from build123d import *

# Parameters (mm, degrees)
F1_W          = 62.5
F1_H          = 102.5
F1_W_2        = 57.5
F1_H_2        = 97.5
F2_DEPTH      = 37
F3_W          = 62.5
F3_H          = 102.5
F4_DEPTH      = 2.5
F6_DEPTH      = 2.501
F7_W          = 51
F7_H          = 72
F8_DEPTH      = 1.2
F10_DEPTH     = 2.5
F11_R         = 1.75
F12_DEPTH     = 102.501
F13_T1_DEPTH  = 42.5
F13_T3_DEPTH  = 57.5
F13_T5_DEPTH  = 42.5
F13_T7_DEPTH  = 57.5
F13_T9_DEPTH  = 44.4614347816
F13_T11_DEPTH = 57.9568101466
F13_T13_DEPTH = 40.0817550719
F13_T15_DEPTH = 127.5
F13_T17_DEPTH = 87.5
F14_R         = 1


# Not quite as in the source:
# - a fillet or chamfer that OpenCascade refuses, or shapes differently, is made with other operations: its cross-section is extruded or revolved along the edge and cut away or added


with BuildPart() as f2:
    # F1 (on Top) → F2 (new body)
    with BuildSketch(Plane.XY):
        with Locations((28.75, 48.75)):
            Rectangle(F1_W, F1_H)
        with Locations((28.75, 48.75)):
            Rectangle(F1_W_2, F1_H_2, mode=Mode.SUBTRACT)
    extrude(amount=F2_DEPTH)

    # F3 (on Top) → F4 (join)
    with BuildSketch(Plane.XY):
        with Locations((28.75, 48.75)):
            Rectangle(F3_W, F3_H)
    extrude(amount=F4_DEPTH)

    # F5 (on face) → F6 (cut, through all)
    with BuildSketch(Plane.XY.offset(2.5)):
        with BuildLine():
            ThreePointArc((17.25, 90.5), (16.25, 89.5), (17.25, 88.5))
            Line((17.25, 88.5), (40.25, 88.5))
            ThreePointArc((40.25, 88.5), (41.25, 89.5), (40.25, 90.5))
            Line((40.25, 90.5), (17.25, 90.5))
        make_face()
        with BuildLine():
            ThreePointArc((17.25, 13), (16.25, 12), (17.25, 11))
            Line((17.25, 11), (40.25, 11))
            ThreePointArc((40.25, 11), (41.25, 12), (40.25, 13))
            Line((40.25, 13), (17.25, 13))
        make_face()
    extrude(amount=-F6_DEPTH, mode=Mode.SUBTRACT)

    # F7 (on face) → F8 (cut)
    with BuildSketch(Plane(origin=(0, 0, 0), x_dir=(1, 0, 0), z_dir=(0, 0, -1))):
        with Locations((28.75, -53.5)):
            Rectangle(F7_W, F7_H)
    extrude(amount=-F8_DEPTH, mode=Mode.SUBTRACT)

    # F9 (on face) → F10 (join)
    with BuildSketch(Plane.XY.offset(2.5)):
        Polygon((0, 32.5), (0, 30), (28.5635979803, 46.412179039), (26.5233409817, 47.7398805363), align=None)
        Polygon((26.5233409817, 47.7398805363), (28.5635979803, 46.412179039), (30.6038549789, 47.5844775418), (28.5635979803, 48.912179039), align=None)
        Polygon((30.6038549789, 47.5844775418), (28.5635979803, 46.412179039), (57.5, 27.5817550719), (57.5, 30.0817550719), align=None)
        Polygon((28.5635979803, 48.912179039), (30.6038549789, 47.5844775418), (57.5, 63.0385652184), (57.5, 65.5385652184), align=None)
        Polygon((0, 65), (26.5233409817, 47.7398805363), (28.5635979803, 48.912179039), (0, 67.5), align=None)
    extrude(amount=F10_DEPTH)

    # F11 (on face) → F12 (cut, through all)
    with BuildSketch(Plane(origin=(0, 100, 0), x_dir=(-1, 0, 0), z_dir=(0, 1, 0))):
        with Locations((-14.5, 29.5)):
            Circle(F11_R)
        with Locations((-43, 29.5)):
            Circle(F11_R)
    extrude(amount=-F12_DEPTH, mode=Mode.SUBTRACT)

    # F13: fillet of radius 5 on 12 edges, made by hand

    # F13_s2 → F13_t1 (join)
    with BuildSketch(Plane.XZ.offset(-42.5)):
        with BuildLine():
            ThreePointArc((0, 7.5), (1.4644660941, 3.9644660941), (5, 2.5))
            Line((5, 2.5), (0, 2.5))
            Line((0, 2.5), (0, 7.5))
        make_face()
    extrude(amount=F13_T1_DEPTH)

    # F13_s4 → F13_t3 (join)
    with BuildSketch(Plane.XZ.offset(-77.5)):
        with BuildLine():
            ThreePointArc((0, 7.5), (1.4644660941, 3.9644660941), (5, 2.5))
            Line((5, 2.5), (0, 2.5))
            Line((0, 2.5), (0, 7.5))
        make_face()
    extrude(amount=F13_T3_DEPTH)

    # F13_s6 → F13_t5 (join)
    with BuildSketch(Plane.XZ.offset(-97.5)):
        with BuildLine():
            ThreePointArc((0, 7.5), (1.4644660941, 3.9644660941), (5, 2.5))
            Line((5, 2.5), (0, 2.5))
            Line((0, 2.5), (0, 7.5))
        make_face()
    extrude(amount=F13_T5_DEPTH)

    # F13_s8 → F13_t7 (join)
    with BuildSketch(Plane.YZ):
        with BuildLine():
            ThreePointArc((0, 7.5), (1.4644660941, 3.9644660941), (5, 2.5))
            Line((5, 2.5), (0, 2.5))
            Line((0, 2.5), (0, 7.5))
        make_face()
        with BuildLine():
            ThreePointArc((97.5, 7.5), (96.0355339059, 3.9644660941), (92.5, 2.5))
            Line((92.5, 2.5), (97.5, 2.5))
            Line((97.5, 2.5), (97.5, 7.5))
        make_face()
    extrude(amount=F13_T7_DEPTH)

    # F13_s10 → F13_t9 (join)
    with BuildSketch(Plane.XZ.offset(-97.5)):
        with BuildLine():
            ThreePointArc((57.5, 7.5), (56.0355339059, 3.9644660941), (52.5, 2.5))
            Line((52.5, 2.5), (57.5, 2.5))
            Line((57.5, 2.5), (57.5, 7.5))
        make_face()
    extrude(amount=F13_T9_DEPTH)

    # F13_s12 → F13_t11 (join)
    with BuildSketch(Plane.XZ.offset(-75.5385652184)):
        with BuildLine():
            ThreePointArc((57.5, 7.5), (56.0355339059, 3.9644660941), (52.5, 2.5))
            Line((52.5, 2.5), (57.5, 2.5))
            Line((57.5, 2.5), (57.5, 7.5))
        make_face()
    extrude(amount=F13_T11_DEPTH)

    # F13_s14 → F13_t13 (join)
    with BuildSketch(Plane.XZ.offset(-40.0817550719)):
        with BuildLine():
            ThreePointArc((57.5, 7.5), (56.0355339059, 3.9644660941), (52.5, 2.5))
            Line((52.5, 2.5), (57.5, 2.5))
            Line((57.5, 2.5), (57.5, 7.5))
        make_face()
    extrude(amount=F13_T13_DEPTH)

    # F13_s16 → F13_t15 (cut)
    with BuildSketch(Plane.XZ.offset(-112.5)):
        with BuildLine():
            ThreePointArc((-2.5, 5), (-1.0355339059, 1.4644660941), (2.5, 0))
            Line((2.5, 0), (-2.5, 0))
            Line((-2.5, 0), (-2.5, 5))
        make_face()
        with BuildLine():
            ThreePointArc((60, 5), (58.5355339059, 1.4644660941), (55, 0))
            Line((55, 0), (60, 0))
            Line((60, 0), (60, 5))
        make_face()
    extrude(amount=F13_T15_DEPTH, mode=Mode.SUBTRACT)

    # F13_s18 → F13_t17 (cut)
    with BuildSketch(Plane.YZ.offset(-15)):
        with BuildLine():
            ThreePointArc((100, 5), (98.5355339059, 1.4644660941), (95, 0))
            Line((95, 0), (100, 0))
            Line((100, 0), (100, 5))
        make_face()
        with BuildLine():
            ThreePointArc((-2.5, 5), (-1.0355339059, 1.4644660941), (2.5, 0))
            Line((2.5, 0), (-2.5, 0))
            Line((-2.5, 0), (-2.5, 5))
        make_face()
    extrude(amount=F13_T17_DEPTH, mode=Mode.SUBTRACT)

    # F14
    f14_edges = [f2.edges().sort_by_distance(p)[0] for p in [
        (60, 100, 21),
        (-2.5, 100, 21),
        (-2.5, -2.5, 21),
        (60, -2.5, 21),
        (0, 0, 22.25),
        (57.5, 0, 22.25),
        (57.5, 97.5, 22.25),
        (0, 97.5, 22.25),
        (-1.035534, 98.535534, 1.464466),
        (58.535534, 98.535534, 1.464466),
        (-1.035534, -1.035534, 1.464466),
        (58.535534, -1.035534, 1.464466),
        (56.035534, 1.464466, 3.964466),
        (1.464466, 1.464466, 3.964466),
        (1.464466, 96.035534, 3.964466),
        (56.035534, 96.035534, 3.964466),
    ]]
    fillet(f14_edges, radius=F14_R)


solid = f2.part
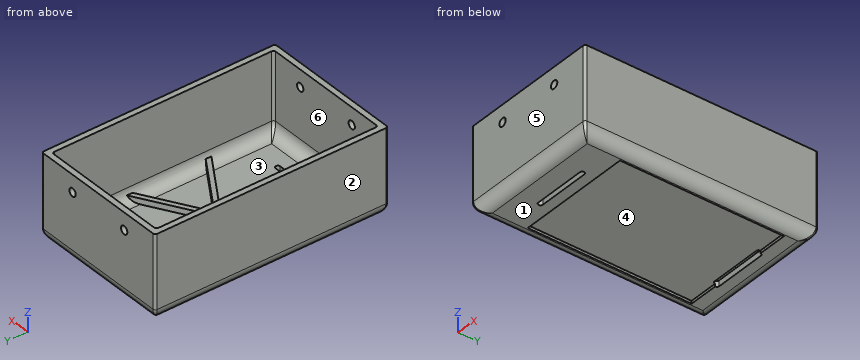
Design review of the part built by this model. Coordinates are the model's own, in mm. Face numbers are marked on the shaded views. A direction names the side the tool comes from. Coordinates: 2 decimals unless noted, no trailing zeros. Order: outer loops, then holes, each group sorted by start corner. A loop starts at its lowest first (then second) coordinate and runs counter-clockwise, first axis right, second up. Notation, with made-up numbers: M 48,16.5 L 79,16.5 A19 cw 79,38.5 Z; hole C 85,21 d1. An arc over 180 degrees is marked long. Use a Markdown table: item, result.
(1) Wall thickness on probe 1 along Y at (x, z) = (49, 3); probe 2 along X at (y, z) = (11, 16.5); probe 3 along Y at (x, z) = (30, 16): over which ranges is each line inside the solid? List them lowest first.
Worked answers:
| item | result |
|---|---|
| probe 1 | y = -2.08 to 2.82, 33.11 to 35.61, 58.15 to 60.65, 94.68 to 99.58 |
| probe 2 | x = -2.5 to 0, 57.5 to 60 |
| probe 3 | y = -2.5 to 0, 97.5 to 100 |
(2) Add section C-C (z = 29.5). Count the separate pieces of the cut face and the enclosed holes in it, then the cut area to 3 significant figures.
Worked answers:
| item | result |
|---|---|
| separate pieces | 4 |
| enclosed holes | 0 |
| area | 765 mm2 |
(3) For P1, Ø10, axis at x = 10.5, y = 22.5, coming from the +Z side; P2, Ø6.5, axis at x = 21, y = 45.5, coming from the +Z side; P3, Ø0.8, axis at x = 32, z = 1.5, coming from the +Y side, all flat-tipped, find the tip position at first contact; note any pin that passes through.
Worked answers:
| item | result |
|---|---|
| P1 | stops at z = 2.5 |
| P2 | stops at z = 5 |
| P3 | stops at y = 98.92 |
(4) For the marked faces 4, 5 and 6, list the 3-axis set-ups (+Z, -Z, +X, -X, +Y, -Y) from which the entire face can be reached by the end or side of a thin tool; tool diameter is ignored.
Worked answers:
| item | result |
|---|---|
| face 4 | -Z |
| face 5 | +Z, -Z, +X, -X, -Y |
| face 6 | +Z |
(5) Add section A-A (z = 34.5). Give the boundary of the cut face in (x, y).
Worked answers:
| item | result |
|---|---|
| outline | M -2.5,-1.5 A1 ccw -1.5,-2.5 L 59,-2.5 A1 ccw 60,-1.5 L 60,99 A1 ccw 59,100 L -1.5,100 A1 ccw -2.5,99 Z; hole M 0,1 A1 ccw 1,0 L 56.5,0 A1 ccw 57.5,1 L 57.5,96.5 A1 ccw 56.5,97.5 L 1,97.5 A1 ccw 0,96.5 Z |
(6) Add section B-B (y = 82). Give the boundary of the cut face in (x, z), then the cut area to 3 significant figures.
Worked answers:
| item | result |
|---|---|
| outline | M -2.5,5 A5 ccw 2.5,0 L 3.25,0 L 3.25,1.2 L 54.25,1.2 L 54.25,0 L 55,0 A5 ccw 60,5 L 60,37 L 57.5,37 L 57.5,7.5 A5 cw 52.5,2.5 L 5,2.5 A5 cw 0,7.5 L 0,37 L -2.5,37 Z |
| area | 268 mm2 |
(7) Draft analysis for pull direction X (two halves, no side actions). For the marked faces 1, 2 and 3, state which applies: released by +X, released by -X, zero draft, split by the parting line, or undercut.
Worked answers:
| item | result |
|---|---|
| face 1 | zero draft |
| face 2 | released by -X |
| face 3 | undercut |
